Build history of the part. All positions in model axes, mm. Round coordinates to 2 decimals unless told otherwise and drop trailing zeros. Write each loop counter-clockwise with the first axis right and the second up, starting at its lowest first coordinate (ties: lowest second). Pieces come first, ordered by that corner, then holes.
Item 1: Band-saw the part on A-A, the plane x = 40. Write the cut outline in (y, z) (3 decimals), then the cut area to 3 significant figures.
Item 2: Band-saw the part on B-B, the plane x = -55. Write the cut outline in (y, z), then the cut area to 3 significant figures.
Item 3: Drop flat-ended pins along their axis: pin 1 Ø3 at (x, y) = (-51.5, 8.5) entering from -Z; pin 2 Ø1.5 at (y, z) = (24.5, -1.5) entering from -X; pin 3 Ø1.5 at (x, z) = (3.5, -28) entering from +Y. Give the stop position or say it passes through.
Item 4: Mould opens along Y. For faces 1 (the flat face through (-1, -59, -35)), 2 (the cylindrical face through (72.5, -40.2, 3)) say: +Y half, -Y half, draft (parallel to the pull), parting line (faces both ways), or undercut.
Item 5: Band-saw the part on C-C, the plane y = -15. Write the cut outline in (x, z) (3 decimals), then the cut area to 3 significant figures.
Item 6: Wall check: probe 1 along Y at (x, z) = (-40, 4) (3 decimals); probe 2 along Z at (x, y) = (-55, -58.75); probe 3 along Y at (x, z) = (-15, 1.85) (3 decimals). Give the ranges that are in metal, low to high.
Item 7: Band-saw the part on D-D, the plane x = 0. Write the cut outline in (y, z) (3 decimals), then the cut area to 3 significant figures.
```python
from build123d import *

# Parameters (mm, degrees)
SKETCH_W      = 152
SKETCH_H      = 102
SKETCH_R      = 2.625
PAD_DEPTH     = 6
SKETCH001_W   = 152
SKETCH001_H   = 41
SKETCH001_R   = 8
SKETCH001_R_2 = 2.125
PAD001_DEPTH  = 6
FILLET_R      = 1.25


with BuildPart() as part:
    # Sketch → Pad (new body)
    with BuildSketch(Plane.XY):
        with Locations((0, -5)):
            Rectangle(SKETCH_W, SKETCH_H)
        with Locations((-70, 41)):
            Circle(SKETCH_R, mode=Mode.SUBTRACT)
        with Locations((-40, 41)):
            Circle(SKETCH_R, mode=Mode.SUBTRACT)
        with Locations((-70, 15)):
            Circle(SKETCH_R, mode=Mode.SUBTRACT)
        with Locations((-40, 15)):
            Circle(SKETCH_R, mode=Mode.SUBTRACT)
        with Locations((-70, -15)):
            Circle(SKETCH_R, mode=Mode.SUBTRACT)
        with Locations((-40, -15)):
            Circle(SKETCH_R, mode=Mode.SUBTRACT)
        with Locations((-70, -41)):
            Circle(SKETCH_R, mode=Mode.SUBTRACT)
        with Locations((-40, -41)):
            Circle(SKETCH_R, mode=Mode.SUBTRACT)
        with Locations((40, 41)):
            Circle(SKETCH_R, mode=Mode.SUBTRACT)
        with Locations((70, 41)):
            Circle(SKETCH_R, mode=Mode.SUBTRACT)
        with Locations((40, 15)):
            Circle(SKETCH_R, mode=Mode.SUBTRACT)
        with Locations((70, 15)):
            Circle(SKETCH_R, mode=Mode.SUBTRACT)
        with Locations((40, -15)):
            Circle(SKETCH_R, mode=Mode.SUBTRACT)
        with Locations((70, -15)):
            Circle(SKETCH_R, mode=Mode.SUBTRACT)
        with Locations((40, -41)):
            Circle(SKETCH_R, mode=Mode.SUBTRACT)
        with Locations((70, -41)):
            Circle(SKETCH_R, mode=Mode.SUBTRACT)
        Circle(SKETCH_R, mode=Mode.SUBTRACT)
        with Locations((-15, 15)):
            Circle(SKETCH_R, mode=Mode.SUBTRACT)
        with Locations((15, 15)):
            Circle(SKETCH_R, mode=Mode.SUBTRACT)
        with Locations((-15, -15)):
            Circle(SKETCH_R, mode=Mode.SUBTRACT)
        with Locations((15, -15)):
            Circle(SKETCH_R, mode=Mode.SUBTRACT)
    extrude(amount=PAD_DEPTH)

    # Sketch001 → Pad001 (new body)
    with BuildSketch(Plane.XZ.offset(56)):
        with Locations((0, -14.5)):
            Rectangle(SKETCH001_W, SKETCH001_H)
        with Locations((0, -16)):
            Circle(SKETCH001_R, mode=Mode.SUBTRACT)
        with Locations((-55, -15)):
            Circle(SKETCH001_R, mode=Mode.SUBTRACT)
        with Locations((55, -15)):
            Circle(SKETCH001_R, mode=Mode.SUBTRACT)
        with Locations((-11.313708, -4.686292)):
            Circle(SKETCH001_R_2, mode=Mode.SUBTRACT)
        with Locations((11.313708, -4.686292)):
            Circle(SKETCH001_R_2, mode=Mode.SUBTRACT)
        with Locations((-16, -16)):
            Circle(SKETCH001_R_2, mode=Mode.SUBTRACT)
        with Locations((16, -16)):
            Circle(SKETCH001_R_2, mode=Mode.SUBTRACT)
        with Locations((-11.313708, -27.313708)):
            Circle(SKETCH001_R_2, mode=Mode.SUBTRACT)
        with Locations((11.313708, -27.313708)):
            Circle(SKETCH001_R_2, mode=Mode.SUBTRACT)
    extrude(amount=PAD001_DEPTH)

    # Fillet
    fillet_edges = [part.edges().sort_by_distance(p)[0] for p in [
        (0, -56, 0),
    ]]
    fillet(fillet_edges, radius=FILLET_R)


solid = part.part
```
Results:
1. outline: (-62, -35) - (-56, -35) - (-56, -1.25) arc R1.25 cw to (-54.75, 0) - (-43.625, 0) - (-43.625, 6) - (-62, 6) - close; (-38.375, 0) - (-17.625, 0) - (-17.625, 6) - (-38.375, 6) - close; (-12.375, 0) - (12.375, 0) - (12.375, 6) - (-12.375, 6) - close; (17.625, 0) - (38.375, 0) - (38.375, 6) - (17.625, 6) - close; (43.625, 0) - (46, 0) - (46, 6) - (43.625, 6) - close
1. area: 732 mm2
2. outline: (-62, -35) - (-56, -35) - (-56, -23) - (-62, -23) - close; (-62, -7) - (-56, -7) - (-56, -1.25) arc R1.25 cw to (-54.75, 0) - (46, 0) - (46, 6) - (-62, 6) - close
2. area: 762 mm2
3. pin 1: stops at z = 0
3. pin 2: passes through
3. pin 3: stops at y = -56
4. face 1: draft
4. face 2: undercut
5. outline: (-76, 0) - (-72.625, 0) - (-72.625, 6) - (-76, 6) - close; (-67.375, 0) - (-42.625, 0) - (-42.625, 6) - (-67.375, 6) - close; (-37.375, 0) - (-17.625, 0) - (-17.625, 6) - (-37.375, 6) - close; (-12.375, 0) - (12.375, 0) - (12.375, 6) - (-12.375, 6) - close; (17.625, 0) - (37.375, 0) - (37.375, 6) - (17.625, 6) - close; (42.625, 0) - (67.375, 0) - (67.375, 6) - (42.625, 6) - close; (72.625, 0) - (76, 0) - (76, 6) - (72.625, 6) - close
5. area: 723 mm2
6. probe 1: y = -62 to -43.625, -38.375 to -17.625, -12.375 to 12.375, 17.625 to 38.375, 43.625 to 46
6. probe 2: z = -35 to -23, -7 to 6
6. probe 3: y = -62 to -17.625, -12.375 to 12.375, 17.625 to 46
7. outline: (-62, -35) - (-56, -35) - (-56, -24) - (-62, -24) - close; (-62, -8) - (-56, -8) - (-56, -1.25) arc R1.25 cw to (-54.75, 0) - (-2.625, 0) - (-2.625, 6) - (-62, 6) - close; (2.625, 0) - (46, 0) - (46, 6) - (2.625, 6) - close
7. area: 731 mm2
